Check sheet for the modelled part. Datum: model origin and axes. Units: mm. A direction names the side the tool comes from. Give positions to 0.01 mm unless a question says otherwise; leave off trailing zeros. Write each loop counter-clockwise with the first axis right and the second up, starting at its lowest first coordinate (ties: lowest second). Pieces come first, ordered by that corner, then holes. Notation, with made-up numbers: (22, 50) -> (77, 50) arc R19 ccw to (77, 61) -> close; hole circle Ø2 at (-15.5, 16.25). An arc over 180 degrees is marked (long way). Return JSON: item names as keys, results as strings.
from build123d import *

# Parameters (mm, degrees)
SKETCH1_W             = 88.9
SKETCH1_H             = 266.7
SKETCH1_R             = 20.6375
BOSS_EXTRUDE1_DEPTH   = 0.4
BOSS_EXTRUDE1_2_DEPTH = 0.4
SKETCH2_W             = 2.54
SKETCH2_H             = 30.48
BOSS_EXTRUDE2_DEPTH   = 0.4


with BuildPart() as part:
    # Sketch1 → Boss-Extrude1 (new body)
    with BuildSketch(Plane(origin=(0, 0, 0), x_dir=(1, 0, 0), z_dir=(0, 1, 0))):
        with Locations((26.9875, -76.2)):
            Rectangle(SKETCH1_W, SKETCH1_H)
        with Locations(Location((26.9875, -44.45, 0), (0, 0, 270))):
            Circle(SKETCH1_R, mode=Mode.SUBTRACT)
        Polygon((10.4775, -162.651716191), (10.4775, -200.025), (1.5875, -200.025), (1.5875, -149.225), (10.4775, -149.225), (43.4975, -186.598283809), (43.4975, -149.225), (52.3875, -149.225), (52.3875, -200.025), (43.4975, -200.025), align=None, mode=Mode.SUBTRACT)
        Polygon((31.4325, 0), (22.5425, 0), (8.89, 29.583775771), (8.89, 0), (0, 0), (0, 50.8), (8.89, 50.8), (26.9875, 11.584297234), (45.085, 50.8), (53.975, 50.8), (53.975, 0), (45.085, 0), (45.085, 29.583775771), align=None, mode=Mode.SUBTRACT)
        with BuildLine():
            ThreePointArc((61.475168351, -31.75), (-9.764224698, -44.45), (61.475168351, -57.15))
            Line((61.475168351, -57.15), (52.585168351, -57.15))
            ThreePointArc((52.585168351, -57.15), (-1.5875, -44.45), (52.585168351, -31.75))
            Line((52.585168351, -31.75), (61.475168351, -31.75))
        make_face(mode=Mode.SUBTRACT)
        with BuildLine():
            Line((1.5875, -88.9), (37.1475, -88.9))
            ThreePointArc((37.1475, -88.9), (52.3875, -104.14), (37.1475, -119.38))
            Line((37.1475, -119.38), (51.375717176, -139.7))
            Line((51.375717176, -139.7), (40.523031082, -139.7))
            Line((40.523031082, -139.7), (26.294813906, -119.38))
            Line((26.294813906, -119.38), (10.4775, -119.38))
            Line((10.4775, -119.38), (10.4775, -139.7))
            Line((10.4775, -139.7), (1.5875, -139.7))
            Line((1.5875, -139.7), (1.5875, -88.9))
        make_face(mode=Mode.SUBTRACT)
    extrude(amount=BOSS_EXTRUDE1_DEPTH)



with BuildPart() as body_2:
    # Sketch1 → Boss-Extrude1 2 (new body)
    with BuildSketch(Plane(origin=(0, 0, 0), x_dir=(1, 0, 0), z_dir=(0, 1, 0))):
        with BuildLine():
            ThreePointArc((37.1475, -97.79), (43.4975, -104.14), (37.1475, -110.49))
            Line((37.1475, -110.49), (10.4775, -110.49))
            Line((10.4775, -110.49), (10.4775, -97.79))
            Line((10.4775, -97.79), (37.1475, -97.79))
        make_face()
    extrude(amount=BOSS_EXTRUDE1_2_DEPTH)


with BuildPart() as part_1:
    add(part.part)

    add(body_2.part)  # Boss-Extrude2 merges body 2
    # Sketch2 → Boss-Extrude2 (add)
    with BuildSketch(Plane(origin=(0, 0.4, 0), x_dir=(1, 0, 0), z_dir=(0, 1, 0))):
        with Locations((25.024813906, -104.14)):
            Rectangle(SKETCH2_W, SKETCH2_H)
    extrude(amount=-BOSS_EXTRUDE2_DEPTH)


solid = part_1.part
(1) Set-up check for faces 1 (the flat face through (17.81, 0.2, -31.47)), 2 (the flat face through (26, 0, 104)): record each of +Z, -Z, +X, -X, +Y, -Y from which the full face is reachable in a straight line by a thin tool's end or side.
Reply:
{"face 1": "+Y, -Y", "face 2": "+Z, -Z, +X, -X, -Y"}
(2) Cross-section at B-B on x = -4. Enter the section's corners in (y, z), then the cut area to 3 significant figures.
Reply:
{"outline": "(0, -57.15) -> (0.4, -57.15) -> (0.4, 24.69) -> (0, 24.69) -> close; (0, 64.21) -> (0.4, 64.21) -> (0.4, 209.55) -> (0, 209.55) -> close", "area": "90.9 mm^2"}
(3) Cross-section at D-D on z = 165. Enter the section's corners in (x, y) (1 decimal), then the cut area to 3 significant figures.
Reply:
{"outline": "(-17.5, 0) -> (1.6, 0) -> (1.6, 0.4) -> (-17.5, 0.4) -> close; (10.5, 0) -> (12.6, 0) -> (12.6, 0.4) -> (10.5, 0.4) -> close; (24.4, 0) -> (43.5, 0) -> (43.5, 0.4) -> (24.4, 0.4) -> close; (52.4, 0) -> (71.4, 0) -> (71.4, 0.4) -> (52.4, 0.4) -> close", "area": "23.7 mm^2"}
(4) Release check for a two-part mould opening along Z. For faces 3 (the flat face through (38.354, 0.197, -14.999)), 4 (the flat face through (26, 0.4, 104)), 5 (the cylindrical face through (43.496, 0.197, 104)) record: pulls with the +Z half, pulls with the -Z half, needs draft (parallel to the pull), parting line crosses it, or undercut.
Reply:
{"face 3": "undercut", "face 4": "needs draft", "face 5": "undercut"}
(5) Cross-section at C-C on y = 0.1. State how many separate pieces and enclosed holes the cut face has, then the cut area to 3 significant figures.
Reply:
{"separate pieces": "1", "enclosed holes": "6", "area": "16,500 mm^2"}
(6) Depth check by flat-ended pin: pin 1 Ø3 at (x, z) = (4, 129) entering from -Y. Enter the tip coordinate at first touch or a pass-through.
Reply:
{"pin 1": "through"}
(7) Cross-section at A-A on z = 104.14. Enter the section's corners in (x, y), then the cut area to 3 significant figures.
Reply:
{"outline": "(-17.46, 0) -> (1.59, 0) -> (1.59, 0.4) -> (-17.46, 0.4) -> close; (10.48, 0) -> (43.5, 0) -> (43.5, 0.4) -> (10.48, 0.4) -> close; (52.39, 0) -> (71.44, 0) -> (71.44, 0.4) -> (52.39, 0.4) -> close", "area": "28.4 mm^2"}
(8) Thickness scan on L1, parallel to X at y = 0.35, z = 103.5; L2, parallel to Z at x = 1.5, y = 0.15; L3, parallel to X at y = 0.15, z = 178. Record the ranges inside material, lowest first.
Reply:
{"L1": "-17.46 to 1.59, 10.48 to 43.47, 52.37 to 71.44", "L2": "-57.15 to -50.8, 0 to 17.97, 31.53 to 57.37, 70.93 to 209.55", "L3": "-17.46 to 1.59, 10.48 to 24.04, 35.9 to 43.5, 52.39 to 71.44"}
